from build123d import *

# Parameters (mm, degrees)
F0_R     = 3.175
F1_DEPTH = 25.4
F2_R     = 5.08
F3_R     = 5.08


with BuildPart() as f1:
    # F0 (on Front) → F1 (new body)
    with BuildSketch(Plane.XZ):
        with BuildLine():
            Line((-31.75, 0), (-19.05, 0))
            ThreePointArc((-19.05, 0), (-5.579616, 5.579616), (0, 19.05))
            ThreePointArc((0, 19.05), (-11.27287, 36.440191), (-31.75, 33.249032))
            Line((-31.75, 33.249032), (-31.75, 0))
        make_face()
        with Locations((-19.05, 19.05)):
            Circle(F0_R, mode=Mode.SUBTRACT)
        with BuildLine():
            ThreePointArc((-31.75, 33.249032), (-11.27287, 36.440191), (0, 19.05))
            ThreePointArc((0, 19.05), (-8.752664, 46.362383), (-31.75, 63.5))
            ThreePointArc((-31.75, 63.5), (-26.160526, 48.374516), (-31.75, 33.249032))
        make_face()
    extrude(amount=F1_DEPTH)

    # F2
    f2_edges = [f1.edges().sort_by_distance(p)[0] for p in [
        (-31.75, -25.4, 16.624516),
        (-25.4, -25.4, 0),
    ]]
    fillet(f2_edges, radius=F2_R)

    # F3
    f3_edges = [f1.edges().sort_by_distance(p)[0] for p in [
        (-31.75, 0, 16.624516),
        (-25.4, 0, 0),
    ]]
    fillet(f3_edges, radius=F3_R)


solid = f1.part
Model file for the job. Use its own axes, mm. A direction names the side the tool comes from. Round coordinates to 2 decimals unless told otherwise and drop trailing zeros. Order: outer loops, then holes, each group sorted by start corner. A loop starts at its lowest first (then second) coordinate and runs counter-clockwise, first axis right, second up.
(1) Pin check, flat tips, straight feed: pin 1 (12 mm diameter, centred on y = -9, z = 46.5, fed in from +X); pin 2 (10 mm diameter, centred on y = -15.5, z = 53.5, fed in from +X); pin 3 (4 mm diameter, centred on x = -3.5, z = 24, fed in from +Y); pin 4 (6 mm diameter, centred on x = -16, y = -6, fed in from +Z). Stop position of each tip, or through.
(2) Drill centre lines: line 1 (Z direction, x = -19.05, y = -10.5) (3 decimals); line 2 (Y direction, x = -27, z = 34); line 3 (Z direction, x = -18, y = -3.5). Where is each one in solid material? Low to high.
(3) Pull direction Z, two halves, no side cores. Call faces 4 (the face through (-5.73, -12.59, 5.43)), 5 (the face through (-19, -25.4, 25)), 6 (the face through (-26.16, -12.52, 48.61)), 7 (the face through (-17.585, -12.522, 16.233)): released by +Z, released by -Z, zero draft, split by the parting line, or undercut.
(4) 3-axis set-ups, long thin cutter, end or side, ignore diameter. For faces 1 (the face through (-30.301, -23.872, 21.462)), 2 (the face through (-30.301, -1.528, 21.462)), 3 (the face through (-23.9, -23.872, 1.449)): which of +Z, -Z, +X, -X, +Y, -Y reach the whole face in a straight line?
(5) Band-saw the part on A-A (y = -8.75). List the corners of the cut face in (x, z) (3 decimals).
Verdict:
1. pin 1: stops at x = -5.18
1. pin 2: stops at x = -10.37
1. pin 3: stops at y = 0
1. pin 4: stops at z = 56.79
2. line 1: z = 0 to 15.875, 22.225 to 56.831
2. line 2: y = -25.39 to -0.01
2. line 3: z = 0.28 to 16.05, 22.05 to 55.71
3. face 4: released by -Z
3. face 5: zero draft
3. face 6: undercut
3. face 7: undercut
4. face 1: -Z, -X, -Y
4. face 2: -Z, -X, +Y
4. face 3: -Z, +X, -X, -Y
5. outline: (-31.75, 0) - (-19.05, 0) arc R19.05 ccw to (0, 19.05) arc R46.99 ccw to (-31.75, 63.5) arc R23.26 cw to (-31.75, 33.249) - close; hole circle Ø6.35 at (-19.05, 19.05)
